```python
from build123d import *

# Parameters (mm, degrees)
BOSS_EXTRU_1_DEPTH      = 3
ENL_V_MAT_EXTRU_1_DEPTH = 58.384666942


with BuildPart() as part:
    # Esquisse1 → Boss.-Extru.1 (new body)
    with BuildSketch(Plane.XY):
        Polygon((-5, -25), (-5, -28), (5, -28), (5, -25), (20, -25), (20, 15), (5, 15), (5, 18), (-5, 18), (-5, 15), (-10, 15), (-10, -25), align=None)
    extrude(amount=BOSS_EXTRU_1_DEPTH)

    # Symétrie1: part across plane


with BuildPart() as part_1:
    add(part.part)
    add(part.part.mirror(Plane(origin=(20, 15, 3), x_dir=(0, 0, 1), z_dir=(-1, 0, 0))))

    # Esquisse2 → Enlèv. mat.-Extru.1 (cut, through all)
    with BuildSketch(Plane.XY.offset(3)):
        with BuildLine():
            Line((5, 7), (35, 7))
            ThreePointArc((35, 7), (38.535533906, 5.535533906), (40, 2))
            Line((40, 2), (40, -12))
            ThreePointArc((40, -12), (38.535533906, -15.535533906), (35, -17))
            Line((35, -17), (5, -17))
            ThreePointArc((5, -17), (1.464466094, -15.535533906), (0, -12))
            Line((0, -12), (0, 2))
            ThreePointArc((0, 2), (1.464466094, 5.535533906), (5, 7))
        make_face()
    extrude(amount=-ENL_V_MAT_EXTRU_1_DEPTH, mode=Mode.SUBTRACT)


solid = part_1.part
```
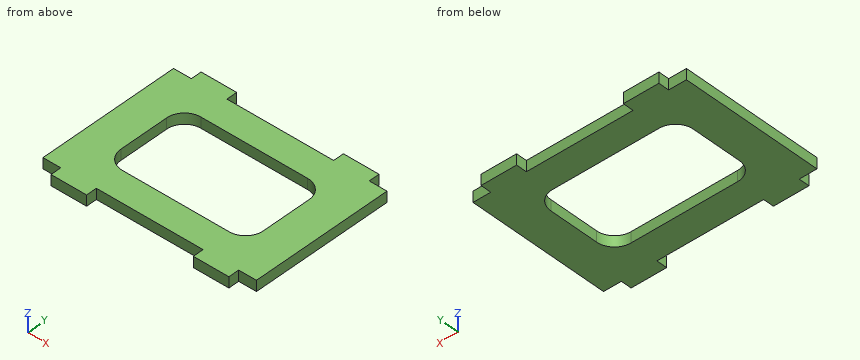
Part model, mm, in its own coordinate system. Round coordinates to 2 decimals unless told otherwise and drop trailing zeros. Loops run counter-clockwise (first coordinate to the right, second up) from the corner with the lowest first, then second, coordinate; pieces in that order, holes last. Notation, with made-up numbers: (17.25, 41.25) -> (76.25, 41.25) arc R23 ccw to (76.25, 59.25) -> close; hole circle Ø8 at (79.5, 46). An arc over 180 degrees is marked (long way). Use CSV: the item, a comma, the result in double quotes. Start each with the question number.
1) Cut at B-B, the plane z = 2. Write the cut outline in (x, y), plus the area to 3 significant figures.
2) Drop flat-ended pins along their axis: P1, Ø0.9, axis at x = 47.5, z = 1, coming from the -Y side; P2, Ø1.5, axis at x = 27.5, z = 2, coming from the +Y side; P3, Ø1.5, axis at y = 16, z = 1.5, coming from the -X side. Give the stop position or say it passes through.
3) Cut at A-A, the plane x = 28.5. Write the cut outline in (y, z), plus the area to 3 significant figures.
4) Wall check: L1, parallel to Y at x = 14.5, z = 0.4; L2, parallel to X at y = -26, z = 1.1; L3, parallel to X at y = 0, z = 0.65. Give the ranges that are in metal, low to high. Write a range as [from, to].
5) Cut at C-C, the plane y = -5. Write the cut outline in (x, z).
Determined:
1,outline,"(-10, -25) -> (-5, -25) -> (-5, -28) -> (5, -28) -> (5, -25) -> (35, -25) -> (35, -28) -> (45, -28) -> (45, -25) -> (50, -25) -> (50, 15) -> (45, 15) -> (45, 18) -> (35, 18) -> (35, 15) -> (5, 15) -> (5, 18) -> (-5, 18) -> (-5, 15) -> (-10, 15) -> close; hole (0, -12) arc R5 ccw to (5, -17) -> (35, -17) arc R5 ccw to (40, -12) -> (40, 2) arc R5 ccw to (35, 7) -> (5, 7) arc R5 ccw to (0, 2) -> close"
1,area,"1,580 mm2"
2,P1,"stops at y = -25"
2,P2,"stops at y = 15"
2,P3,"stops at x = -5"
3,outline,"(-25, 0) -> (-17, 0) -> (-17, 3) -> (-25, 3) -> close; (7, 0) -> (15, 0) -> (15, 3) -> (7, 3) -> close"
3,area,"48.0 mm2"
4,L1,"y = [-25, -17], [7, 15]"
4,L2,"x = [-5, 5], [35, 45]"
4,L3,"x = [-10, 0], [40, 50]"
5,outline,"(-10, 0) -> (0, 0) -> (0, 3) -> (-10, 3) -> close; (40, 0) -> (50, 0) -> (50, 3) -> (40, 3) -> close"
